Part model, mm, in its own coordinate system. A direction names the side the tool comes from. Give positions to 0.01 mm unless a question says otherwise; leave off trailing zeros. Loops run counter-clockwise (first coordinate to the right, second up) from the corner with the lowest first, then second, coordinate; pieces in that order, holes last. Notation, with made-up numbers: (80.5, 67.5) -> (132.5, 67.5) arc R15 ccw to (132.5, 77.5) -> close; hole circle Ø10 at (43, 54). An arc over 180 degrees is marked (long way). Write item = value, one per line.
from build123d import *

# Parameters (mm, degrees)
SKETCH1_W           = 31.75
SKETCH1_H           = 54.61
BOSS_EXTRUDE1_DEPTH = 2.54
SKETCH2_W           = 2.54
SKETCH2_H           = 7.62
SKETCH2_H_2         = 54.61
BOSS_EXTRUDE2_DEPTH = 22.86
SKETCH3_W           = 36.83
SKETCH3_H           = 8.89
BOSS_EXTRUDE3_DEPTH = 25.4
SKETCH4_R           = 1.905
CUT_EXTRUDE1_DEPTH  = 2.54
SKETCH5_W           = 10.16
SKETCH5_H           = 3.175
BOSS_EXTRUDE4_DEPTH = 6.35
SKETCH6_W           = 10.16
SKETCH6_H           = 3.175
BOSS_EXTRUDE5_DEPTH = 6.35
SKETCH7_R           = 1.4224
CUT_EXTRUDE2_DEPTH  = 84.214078887


with BuildPart() as part:
    # Sketch1 → Boss-Extrude1 (new body)
    with BuildSketch(Plane(origin=(0, 0, 0), x_dir=(1, 0, 0), z_dir=(0, 1, 0))):
        with Locations((15.875, 27.305)):
            Rectangle(SKETCH1_W, SKETCH1_H)
    extrude(amount=BOSS_EXTRUDE1_DEPTH)

    # Sketch2 → Boss-Extrude2 (add)
    with BuildSketch(Plane(origin=(0, 0, 0), x_dir=(1, 0, 0), z_dir=(0, 1, 0))):
        with Locations((33.02, 2.54)):
            Rectangle(SKETCH2_W, SKETCH2_H)
        with Locations((33.02, 52.07)):
            Rectangle(SKETCH2_W, SKETCH2_H)
        with Locations((-1.27, 27.305)):
            Rectangle(SKETCH2_W, SKETCH2_H_2)
    extrude(amount=BOSS_EXTRUDE2_DEPTH)

    # Sketch3 → Boss-Extrude3 (add)
    with BuildSketch(Plane.XZ):
        with Locations((15.875, -4.445)):
            Rectangle(SKETCH3_W, SKETCH3_H)
        with Locations((15.875, -50.165)):
            Rectangle(SKETCH3_W, SKETCH3_H)
    extrude(amount=BOSS_EXTRUDE3_DEPTH)

    # Sketch4 → Cut-Extrude1 (cut)
    with BuildSketch(Plane(origin=(34.29, 0, 0), x_dir=(0, 0, -1), z_dir=(1, 0, 0))):
        with Locations((1.85, 17.967840319)):
            Circle(SKETCH4_R)
        with Locations((1.85, 7.967840319)):
            Circle(SKETCH4_R)
        with Locations((52.76, 17.967840319)):
            Circle(SKETCH4_R)
        with Locations((52.76, 7.967840319)):
            Circle(SKETCH4_R)
    extrude(amount=-CUT_EXTRUDE1_DEPTH, mode=Mode.SUBTRACT)

    # Sketch5 → Boss-Extrude4 (add)
    with BuildSketch(Plane(origin=(0, 0, -54.61), x_dir=(-1, 0, 0), z_dir=(0, 0, -1))):
        with Locations((-29.21, -23.8125)):
            Rectangle(SKETCH5_W, SKETCH5_H)
        with Locations((-2.54, -23.8125)):
            Rectangle(SKETCH5_W, SKETCH5_H)
    extrude(amount=BOSS_EXTRUDE4_DEPTH)

    # Sketch6 → Boss-Extrude5 (add)
    with BuildSketch(Plane.XY):
        with Locations((29.21, -23.8125)):
            Rectangle(SKETCH6_W, SKETCH6_H)
        with Locations((2.54, -23.8125)):
            Rectangle(SKETCH6_W, SKETCH6_H)
    extrude(amount=BOSS_EXTRUDE5_DEPTH)

    # Sketch7 → Cut-Extrude2 (cut, through all)
    with BuildSketch(Plane(origin=(0, -22.225, 0), x_dir=(1, 0, 0), z_dir=(0, 1, 0))):
        with Locations(Location((29.21, 57.785, 0), (0, 0, 270))):
            Circle(SKETCH7_R)
        with Locations(Location((2.54, 57.785, 0), (0, 0, 270))):
            Circle(SKETCH7_R)
        with Locations(Location((2.54, -3.175, 0), (0, 0, 270))):
            Circle(SKETCH7_R)
        with Locations(Location((29.21, -3.175, 0), (0, 0, 270))):
            Circle(SKETCH7_R)
    extrude(amount=-CUT_EXTRUDE2_DEPTH, mode=Mode.SUBTRACT)


solid = part.part
1) Drill centre lines: line 1 along Y through (x, z) = (32.5, -1.85); line 2 along Z through (x, y) = (32, -15.5); line 3 along Z through (x, y) = (2, -24). Where is each one in solid material? Low to high. Write a range as [from, to].
Resolved:
line_1 = [-25.4, 6.06], [9.87, 16.06], [19.87, 22.86]
line_2 = [-54.61, -45.72], [-8.89, 0]
line_3 = [-60.96, -59.1], [-56.47, -45.72], [-8.89, 1.86], [4.49, 6.35]
2) Drop flat-ended pins along their axis: P1, Ø12, axis at x = 21, y = -2, coming from the +Z side; P2, Ø2, axis at x = 32.5, z = -46.5, coming from the +Y side; P3, Ø1.9, axis at x = 4.5, z = -58.5, coming from the +Y side (3 decimals). Give the stop position or say it passes through.
Resolved:
P1 = 0
P2 = 2.54
P3 = -22.225
3) Slice it at A-A, the plane z = -52.76. List the corners of the cut face in (x, y), and give its area (3 significant figures).
Resolved:
outline = (-2.54, -25.4) -> (34.29, -25.4) -> (34.29, 6.06) -> (31.75, 6.06) -> (31.75, 2.54) -> (0, 2.54) -> (0, 22.86) -> (-2.54, 22.86) -> close; (31.75, 9.87) -> (34.29, 9.87) -> (34.29, 16.06) -> (31.75, 16.06) -> close; (31.75, 19.87) -> (34.29, 19.87) -> (34.29, 22.86) -> (31.75, 22.86) -> close
area = 1,110 mm²
4) Which spindle directions (+Z, -Z, +X, -X, +Y, -Y) get a long thin tool onto all of the face, cutting with end or side? Do faces 1 (the face through (24.13, -24, -58)), 2 (the face through (4, -22.225, 2)), 3 (the face through (33, 11, -6.35)), 4 (the face through (33, 11, -55.88)), 5 (the face through (33.038, 8.052, -50.857)). Say none if no direction does.
Resolved:
face_1 = -Z, +Y, -Y
face_2 = +Z, +X, -X, +Y
face_3 = +X, +Y
face_4 = -Z, +X, -X, +Y
face_5 = +X
5) Slice it at B-B, the plane x = 32.5. List the corners of the cut face in (y, z) (3 decimals).
Resolved:
outline = (-25.4, -60.96) -> (-22.225, -60.96) -> (-22.225, -54.61) -> (0, -54.61) -> (0, -55.88) -> (22.86, -55.88) -> (22.86, -48.26) -> (0, -48.26) -> (0, -45.72) -> (-25.4, -45.72) -> close; (-25.4, -8.89) -> (0, -8.89) -> (0, -6.35) -> (22.86, -6.35) -> (22.86, 1.27) -> (0, 1.27) -> (0, 0) -> (-22.225, 0) -> (-22.225, 6.35) -> (-25.4, 6.35) -> close; hole circle Ø3.81 at (7.968, -52.76); hole circle Ø3.81 at (7.968, -1.85); hole circle Ø3.81 at (17.968, -52.76); hole circle Ø3.81 at (17.968, -1.85)
6) Slice it at C-C, the plane y = 4.5. List the corners of the cut face in (x, z), and give its area (3 significant figures).
Resolved:
outline = (-2.54, -54.61) -> (0, -54.61) -> (0, 0) -> (-2.54, 0) -> close; (31.75, -55.88) -> (34.29, -55.88) -> (34.29, -48.26) -> (31.75, -48.26) -> close; (31.75, -6.35) -> (34.29, -6.35) -> (34.29, 1.27) -> (31.75, 1.27) -> close
area = 177 mm²
7) Slice it at D-D, the plane y = -11.5. List the corners of the cut face in (x, z), and give its area (3 significant figures).
Resolved:
outline = (-2.54, -54.61) -> (34.29, -54.61) -> (34.29, -45.72) -> (-2.54, -45.72) -> close; (-2.54, -8.89) -> (34.29, -8.89) -> (34.29, 0) -> (-2.54, 0) -> close
area = 655 mm²
8) Pull direction X, two halves, no side cores. Call faces 6 (the face through (34.29, -7, -3)), 7 (the face through (33, 11, -48.26)), 8 (the face through (29.64, -23.79, -56.43)): pulls with the +X half, pulls with the -X half, needs draft (parallel to the pull), parting line crosses it, or undercut.
Resolved:
face_6 = pulls with the +X half
face_7 = needs draft
face_8 = undercut
